```python
from build123d import *

# Parameters (mm, degrees)
F1_DEPTH = 266.7
F3_DEPTH = 533.4


with BuildPart() as f1:
    # F0 (on Top) → F1 (new body)
    with BuildSketch(Plane.XY):
        Polygon((0, 101.6), (-533.4, 101.6), (-431.8, 0), (-533.4, -101.6), (0, -101.6), (-101.6, 0), align=None)
    extrude(amount=F1_DEPTH)

    # F2 (on Right) → F3 (join)
    with BuildSketch(Plane.YZ):
        Polygon((0, -228.6), (101.6, 0), (-101.6, 0), align=None)
    extrude(amount=-F3_DEPTH)


solid = f1.part
```
Verification items for the finished model (mm, model axes). A direction names the side the tool comes from. Round coordinates to 2 decimals unless told otherwise and drop trailing zeros. Write each loop counter-clockwise with the first axis right and the second up, starting at its lowest first coordinate (ties: lowest second). Pieces come first, ordered by that corner, then holes.
1. Section check A-A on y = 7. Enter the section's corners in (x, z), plus the area to 3 significant figures.
2. Section check C-C on z = 37.5. Enter the section's corners in (x, y).
3. Scan lines: L1, parallel to Y at x = -468, z = 120; L2, parallel to Z at x = -171, y = 33; L3, parallel to Z at x = -294, y = -83. Record each from-to range of solid material in increasing order.
4. Section check B-B on x = -70. Enter the section's corners in (y, z), plus the area to 3 significant figures.
5. Access from +Z, -Z, +X, -X, +Y, -Y to the whole of each face (thin tool, end or side, straight path). Record for faces 4 (the flat face through (-483.3, 51.5, 131.5)), 5 (the flat face through (-270, 1, 266.7)), 6 (the flat face through (-39, 1, 0)).
6. Section check D-D on y = -43. Enter the section's corners in (x, z), plus the area to 3 significant figures.
7. Gauge pin test, flat ends, axial feed: P1, Ø4, axis at y = 37.5, z = 132.5, coming from the -X side; P2, Ø2, axis at x = -381, y = -14, coming from the -Z side; P3, Ø8, axis at x = -317, y = -71, coming from the -Z side. Record the tip position at first contact, or that the pin passes through.
8. Draft check along Y on faces 1 (the flat face through (-50.1, -51.5, 131.5)), 2 (the flat face through (-263, 101.6, 131)), 3 (the flat face through (-533.4, -1, -87)). Enter one of: +Y half, -Y half, draft (parallel to the pull), parting line (faces both ways), or undercut.
Answer:
1. outline: (-533.4, -212.85) - (0, -212.85) - (0, 0) - (-94.6, 0) - (-94.6, 266.7) - (-438.8, 266.7) - (-438.8, 0) - (-533.4, 0) - close
1. area: 205,000 mm2
2. outline: (-533.4, -101.6) - (0, -101.6) - (-101.6, 0) - (0, 101.6) - (-533.4, 101.6) - (-431.8, 0) - close
3. L1: y = -101.6 to -36.2, 36.2 to 101.6
3. L2: z = -154.35 to 266.7
3. L3: z = -41.85 to 266.7
4. outline: (-101.6, 0) - (0, -228.6) - (101.6, 0) - (101.6, 266.7) - (31.6, 266.7) - (31.6, 0) - (-31.6, 0) - (-31.6, 266.7) - (-101.6, 266.7) - close
4. area: 60,600 mm2
5. face 4: +Z, -X
5. face 5: +Z, +X, -X, +Y, -Y
5. face 6: +Z, +X
6. outline: (-533.4, -131.85) - (0, -131.85) - (0, 0) - (-58.6, 0) - (-58.6, 266.7) - (-474.8, 266.7) - (-474.8, 0) - (-533.4, 0) - close
6. area: 181,000 mm2
7. P1: stops at x = -471.3
7. P2: stops at z = -199.35
7. P3: stops at z = -77.85
8. face 1: undercut
8. face 2: +Y half
8. face 3: draft
